from build123d import *

# Parameters (mm, degrees)
SKETCH_1_W          = 237
SKETCH_1_H          = 338
EXTRUDE_1_DEPTH     = 264
SKETCH_2_W          = 197
SKETCH_2_H          = 275
CUT_EXTRUDE_1_DEPTH = 248
SKETCH_3_W          = 237
SKETCH_3_H          = 5
EXTRUDE_2_DEPTH     = 255
EXTRUDE_START       = 70
SKETCH_4_R          = 5
EXTRUDE_3_DEPTH     = 30
SKETCH_6_W          = 338
SKETCH_6_H          = 237
EXTRUDE_6_DEPTH     = 34
FILLET_1_R          = 25
FILLET_2_R          = 10
FILLET_3_R          = 5
FILLET_4_R          = 15
FILLET_5_R          = 15


with BuildPart() as part:
    # 草图1 → 凸台-拉伸1 (new body)
    with BuildSketch(Plane.XY):
        Rectangle(SKETCH_1_W, SKETCH_1_H)
    extrude(amount=-EXTRUDE_1_DEPTH)

    # 草图2 → 切除-拉伸1 (cut)
    with BuildSketch(Plane.XY):
        Rectangle(SKETCH_2_W, SKETCH_2_H)
    extrude(amount=-CUT_EXTRUDE_1_DEPTH, mode=Mode.SUBTRACT)

    # 草图3 → 凸台-拉伸2 (add)
    with BuildSketch(Plane.XY):
        Rectangle(SKETCH_3_W, SKETCH_3_H)
    extrude(amount=-EXTRUDE_2_DEPTH)

    # 草图4 → 凸台-拉伸3 (add)
    with BuildSketch(Plane(origin=(0, 0, 0), x_dir=(1, 0, 0), z_dir=(0, 1, 0)).offset(EXTRUDE_START)):
        with Locations((118.5, 0)):
            Circle(SKETCH_4_R)
    extrude_3 = extrude(amount=EXTRUDE_3_DEPTH)

    # 镜向1: 凸台-拉伸3 across plane
    add(extrude_3.mirror(Plane.ZX))

    # 草图6 → 凸台-拉伸6 (add)
    with BuildSketch(Plane(origin=(59.25, 0, -59.25), x_dir=(0, 1, 0), z_dir=(-0.7071067811865438, 0, 0.7071067811865512))):
        with Locations((0, -200.292153571)):
            Rectangle(SKETCH_6_W, SKETCH_6_H)
    extrude(amount=-EXTRUDE_6_DEPTH)

    # 圆角1
    # the kernel refuses this fillet: 25 mm, written as the material it takes off along each edge
    with BuildSketch(Plane(origin=(118.5, -169, 59.671572875), x_dir=(-1, 0, 0), z_dir=(0, 0, -1))) as fillet_1_piece_1_section:
        with BuildLine():
            CenterArc((FILLET_1_R, FILLET_1_R), FILLET_1_R, 180, 90)
            Line((0, FILLET_1_R), (-FILLET_1_R * 0.02, FILLET_1_R))
            Line((-FILLET_1_R * 0.02, FILLET_1_R), (-FILLET_1_R * 0.02, -FILLET_1_R * 0.02))
            Line((-FILLET_1_R * 0.02, -FILLET_1_R * 0.02), (FILLET_1_R, -FILLET_1_R * 0.02))
            Line((FILLET_1_R, -FILLET_1_R * 0.02), (FILLET_1_R, 0))
        make_face()
    fillet_1_piece_1 = extrude(amount=323.671572875, mode=Mode.PRIVATE)
    fillet_1_piece_1 = split(fillet_1_piece_1, bisect_by=Plane(origin=(179.466338067, -163.404434067, -63.794765192), z_dir=(-0.7071067811865512, 0, -0.7071067811865438)), keep=Keep.TOP, mode=Mode.PRIVATE)
    add(fillet_1_piece_1, mode=Mode.SUBTRACT)
    with BuildSketch(Plane(origin=(-118.5, -169, 0), x_dir=(1, 0, 0), z_dir=(0, 0, -1)), Plane(origin=(-118.5, 169, 0), x_dir=(0, -1, 0), z_dir=(0, 0, -1))) as fillet_1_piece_2:
        with BuildLine():
            CenterArc((FILLET_1_R, -FILLET_1_R), FILLET_1_R, 90, 90)
            Line((0, -FILLET_1_R), (-FILLET_1_R * 0.02, -FILLET_1_R))
            Line((-FILLET_1_R * 0.02, -FILLET_1_R), (-FILLET_1_R * 0.02, FILLET_1_R * 0.02))
            Line((-FILLET_1_R * 0.02, FILLET_1_R * 0.02), (FILLET_1_R, FILLET_1_R * 0.02))
            Line((FILLET_1_R, FILLET_1_R * 0.02), (FILLET_1_R, 0))
        make_face()
    extrude(amount=264, mode=Mode.SUBTRACT)
    with BuildSketch(Plane(origin=(118.5, 169, 59.671572875), x_dir=(0, -1, 0), z_dir=(0, 0, -1))) as fillet_1_piece_3_section:
        with BuildLine():
            CenterArc((FILLET_1_R, FILLET_1_R), FILLET_1_R, 180, 90)
            Line((0, FILLET_1_R), (-FILLET_1_R * 0.02, FILLET_1_R))
            Line((-FILLET_1_R * 0.02, FILLET_1_R), (-FILLET_1_R * 0.02, -FILLET_1_R * 0.02))
            Line((-FILLET_1_R * 0.02, -FILLET_1_R * 0.02), (FILLET_1_R, -FILLET_1_R * 0.02))
            Line((FILLET_1_R, -FILLET_1_R * 0.02), (FILLET_1_R, 0))
        make_face()
    fillet_1_piece_3 = extrude(amount=323.671572875, mode=Mode.PRIVATE)
    fillet_1_piece_3 = split(fillet_1_piece_3, bisect_by=Plane(origin=(179.466338067, 163.404434067, -63.794765192), z_dir=(-0.7071067811865512, 0, -0.7071067811865438)), keep=Keep.TOP, mode=Mode.PRIVATE)
    add(fillet_1_piece_3, mode=Mode.SUBTRACT)
    with BuildSketch(Plane(origin=(284.670093579, -169, 166.170093579), x_dir=(-0.7071067811865512, -1.1368683772161603e-15, -0.7071067811865439), z_dir=(0.7071067811865438, 0, -0.7071067811865512))) as fillet_1_piece_4:
        with BuildLine():
            CenterArc((FILLET_1_R, FILLET_1_R), FILLET_1_R, 180, 90)
            Line((0, FILLET_1_R), (-FILLET_1_R * 0.02, FILLET_1_R))
            Line((-FILLET_1_R * 0.02, FILLET_1_R), (-FILLET_1_R * 0.02, -FILLET_1_R * 0.02))
            Line((-FILLET_1_R * 0.02, -FILLET_1_R * 0.02), (FILLET_1_R, -FILLET_1_R * 0.02))
            Line((FILLET_1_R, -FILLET_1_R * 0.02), (FILLET_1_R, 0))
        make_face()
    extrude(amount=34, mode=Mode.SUBTRACT)
    with BuildSketch(Plane(origin=(74.305826176, -169, 41.365746699), x_dir=(0.7071067811865512, 0, 0.7071067811865439), z_dir=(0.7071067811865438, 0, -0.7071067811865512))) as fillet_1_piece_5_section:
        with BuildLine():
            CenterArc((FILLET_1_R, -FILLET_1_R), FILLET_1_R, 90, 90)
            Line((0, -FILLET_1_R), (-FILLET_1_R * 0.02, -FILLET_1_R))
            Line((-FILLET_1_R * 0.02, -FILLET_1_R), (-FILLET_1_R * 0.02, FILLET_1_R * 0.02))
            Line((-FILLET_1_R * 0.02, FILLET_1_R * 0.02), (FILLET_1_R, FILLET_1_R * 0.02))
            Line((FILLET_1_R, FILLET_1_R * 0.02), (FILLET_1_R, 0))
        make_face()
    fillet_1_piece_5 = extrude(amount=94.5, mode=Mode.PRIVATE)
    fillet_1_piece_5 = split(fillet_1_piece_5, bisect_by=Plane(origin=(118.5, -163.795791277, -7.320817928), z_dir=(1, 0, 0)), keep=Keep.TOP, mode=Mode.PRIVATE)
    add(fillet_1_piece_5, mode=Mode.SUBTRACT)
    with BuildSketch(Plane(origin=(74.305826176, 169, 41.365746699), x_dir=(0.7071067811865512, 0, 0.7071067811865438), z_dir=(0.7071067811865438, 0, -0.7071067811865512))) as fillet_1_piece_6_section:
        with BuildLine():
            CenterArc((FILLET_1_R, FILLET_1_R), FILLET_1_R, 180, 90)
            Line((0, FILLET_1_R), (-FILLET_1_R * 0.02, FILLET_1_R))
            Line((-FILLET_1_R * 0.02, FILLET_1_R), (-FILLET_1_R * 0.02, -FILLET_1_R * 0.02))
            Line((-FILLET_1_R * 0.02, -FILLET_1_R * 0.02), (FILLET_1_R, -FILLET_1_R * 0.02))
            Line((FILLET_1_R, -FILLET_1_R * 0.02), (FILLET_1_R, 0))
        make_face()
    fillet_1_piece_6 = extrude(amount=94.5, mode=Mode.PRIVATE)
    fillet_1_piece_6 = split(fillet_1_piece_6, bisect_by=Plane(origin=(118.5, 163.795791277, -7.320817928), z_dir=(1, 0, 0)), keep=Keep.TOP, mode=Mode.PRIVATE)
    add(fillet_1_piece_6, mode=Mode.SUBTRACT)
    with BuildSketch(Plane(origin=(284.670093579, 169, 166.170093579), x_dir=(-0.7071067811865512, -3.4106051316484808e-15, -0.7071067811865439), z_dir=(0.7071067811865438, 0, -0.7071067811865512))) as fillet_1_piece_7:
        with BuildLine():
            CenterArc((FILLET_1_R, -FILLET_1_R), FILLET_1_R, 90, 90)
            Line((0, -FILLET_1_R), (-FILLET_1_R * 0.02, -FILLET_1_R))
            Line((-FILLET_1_R * 0.02, -FILLET_1_R), (-FILLET_1_R * 0.02, FILLET_1_R * 0.02))
            Line((-FILLET_1_R * 0.02, FILLET_1_R * 0.02), (FILLET_1_R, FILLET_1_R * 0.02))
            Line((FILLET_1_R, FILLET_1_R * 0.02), (FILLET_1_R, 0))
        make_face()
    extrude(amount=34, mode=Mode.SUBTRACT)
    with BuildSketch(Plane(origin=(118.5, -169, 59.671572875), x_dir=(-1, 0, 0), z_dir=(0, 0, -1))) as fillet_1_piece_8a_section:
        with BuildLine():
            CenterArc((FILLET_1_R, FILLET_1_R), FILLET_1_R, 180, 90)
            Line((0, FILLET_1_R), (-FILLET_1_R * 0.02, FILLET_1_R))
            Line((-FILLET_1_R * 0.02, FILLET_1_R), (-FILLET_1_R * 0.02, -FILLET_1_R * 0.02))
            Line((-FILLET_1_R * 0.02, -FILLET_1_R * 0.02), (FILLET_1_R, -FILLET_1_R * 0.02))
            Line((FILLET_1_R, -FILLET_1_R * 0.02), (FILLET_1_R, 0))
        make_face()
    fillet_1_piece_8a = extrude(amount=323.671572875, mode=Mode.PRIVATE)
    fillet_1_piece_8a = split(fillet_1_piece_8a, bisect_by=Plane(origin=(99.013375852, -163.038214912, 16.658197024), z_dir=(0.7071067811865512, 0, 0.7071067811865438)), keep=Keep.TOP, mode=Mode.PRIVATE)
    with BuildSketch(Plane(origin=(74.305826176, -169, 41.365746699), x_dir=(0.7071067811865512, 0, 0.7071067811865439), z_dir=(0.7071067811865438, 0, -0.7071067811865512))) as fillet_1_piece_8b_section:
        with BuildLine():
            CenterArc((FILLET_1_R, -FILLET_1_R), FILLET_1_R, 90, 90)
            Line((0, -FILLET_1_R), (-FILLET_1_R * 0.02, -FILLET_1_R))
            Line((-FILLET_1_R * 0.02, -FILLET_1_R), (-FILLET_1_R * 0.02, FILLET_1_R * 0.02))
            Line((-FILLET_1_R * 0.02, FILLET_1_R * 0.02), (FILLET_1_R, FILLET_1_R * 0.02))
            Line((FILLET_1_R, FILLET_1_R * 0.02), (FILLET_1_R, 0))
        make_face()
    fillet_1_piece_8b = extrude(amount=94.5, mode=Mode.PRIVATE)
    fillet_1_piece_8b = split(fillet_1_piece_8b, bisect_by=Plane(origin=(118.5, -163.038214912, 24.729821031), z_dir=(-1, 0, 0)), keep=Keep.TOP, mode=Mode.PRIVATE)
    fillet_1_piece_8 = fillet_1_piece_8a & fillet_1_piece_8b
    add(fillet_1_piece_8, mode=Mode.SUBTRACT)
    with BuildSketch(Plane(origin=(118.5, 169, 59.671572875), x_dir=(0, -1, 0), z_dir=(0, 0, -1))) as fillet_1_piece_9a_section:
        with BuildLine():
            CenterArc((FILLET_1_R, FILLET_1_R), FILLET_1_R, 180, 90)
            Line((0, FILLET_1_R), (-FILLET_1_R * 0.02, FILLET_1_R))
            Line((-FILLET_1_R * 0.02, FILLET_1_R), (-FILLET_1_R * 0.02, -FILLET_1_R * 0.02))
            Line((-FILLET_1_R * 0.02, -FILLET_1_R * 0.02), (FILLET_1_R, -FILLET_1_R * 0.02))
            Line((FILLET_1_R, -FILLET_1_R * 0.02), (FILLET_1_R, 0))
        make_face()
    fillet_1_piece_9a = extrude(amount=323.671572875, mode=Mode.PRIVATE)
    fillet_1_piece_9a = split(fillet_1_piece_9a, bisect_by=Plane(origin=(99.013375852, 163.038214912, 16.658197024), z_dir=(0.7071067811865512, 0, 0.7071067811865438)), keep=Keep.TOP, mode=Mode.PRIVATE)
    with BuildSketch(Plane(origin=(74.305826176, 169, 41.365746699), x_dir=(0.7071067811865512, 0, 0.7071067811865438), z_dir=(0.7071067811865438, 0, -0.7071067811865512))) as fillet_1_piece_9b_section:
        with BuildLine():
            CenterArc((FILLET_1_R, FILLET_1_R), FILLET_1_R, 180, 90)
            Line((0, FILLET_1_R), (-FILLET_1_R * 0.02, FILLET_1_R))
            Line((-FILLET_1_R * 0.02, FILLET_1_R), (-FILLET_1_R * 0.02, -FILLET_1_R * 0.02))
            Line((-FILLET_1_R * 0.02, -FILLET_1_R * 0.02), (FILLET_1_R, -FILLET_1_R * 0.02))
            Line((FILLET_1_R, -FILLET_1_R * 0.02), (FILLET_1_R, 0))
        make_face()
    fillet_1_piece_9b = extrude(amount=94.5, mode=Mode.PRIVATE)
    fillet_1_piece_9b = split(fillet_1_piece_9b, bisect_by=Plane(origin=(118.5, 163.038214912, 24.729821031), z_dir=(-1, 0, 0)), keep=Keep.TOP, mode=Mode.PRIVATE)
    fillet_1_piece_9 = fillet_1_piece_9a & fillet_1_piece_9b
    add(fillet_1_piece_9, mode=Mode.SUBTRACT)

    # 圆角2
    fillet_2_edges = [part.edges().sort_by_distance(p)[0] for p in [
        (0, -169, -264),
        (118.5, 0, -264),
        (-118.5, 0, -264),
        (0, 169, -264),
        (-111.17766953, 161.67766953, -264),
        (111.17766953, 161.67766953, -264),
        (-111.17766953, -161.67766953, -264),
        (111.17766953, -161.67766953, -264),
    ]]
    fillet(fillet_2_edges, radius=FILLET_2_R)

    # 圆角3
    fillet_3_edges = [part.edges().sort_by_distance(p)[0] for p in [
        (224.919570569, -169, 58.336309448),
        (141.127416998, 0, -25.455844123),
        (224.919570569, 169, 58.336309448),
        (308.711724139, 0, 142.128463018),
        (146.305086528, 161.67766953, -20.278174593),
        (303.53405461, 161.67766953, 136.950793489),
        (303.53405461, -161.67766953, 136.950793489),
        (146.305086528, -161.67766953, -20.278174593),
    ]]
    fillet(fillet_3_edges, radius=FILLET_3_R)

    # 圆角4
    fillet_4_edges = [part.edges().sort_by_distance(p)[0] for p in [
        (98.5, -70, -248),
        (98.5, 137.5, -124),
        (0, -137.5, -248),
        (98.5, -137.5, -124),
        (-98.5, -137.5, -124),
        (0, 137.5, -248),
        (-98.5, 137.5, -124),
        (-98.5, -70, -248),
    ]]
    fillet(fillet_4_edges, radius=FILLET_4_R)

    # 圆角5
    # the kernel refuses this fillet: 15 mm, written as the material it adds along each edge
    with BuildSketch(Plane(origin=(-83.5, 122.5, -233), x_dir=(0, 0, -1), z_dir=(-1, 0, 0))) as fillet_5_piece_1_section:
        Polygon((0, 0), (FILLET_5_R * 1.02, 0), (FILLET_5_R * 1.02, -FILLET_5_R * 1.02), (0, -FILLET_5_R * 1.02), align=None)
    fillet_5_piece_1 = extrude(amount=FILLET_5_R * 1.02, mode=Mode.PRIVATE)
    fillet_5_piece_1 = fillet_5_piece_1 - Plane(origin=(-83.5, 122.5, -233), x_dir=(0, -0.7071067811865475, 0.7071067811865475), z_dir=(-1, 0, 0)) * Sphere(FILLET_5_R, mode=Mode.PRIVATE)
    add(fillet_5_piece_1)
    with BuildSketch(Plane(origin=(83.5, 122.5, -233), x_dir=(0, 0, -1), z_dir=(1, 0, 0))) as fillet_5_piece_2_section:
        Polygon((0, 0), (FILLET_5_R * 1.02, 0), (FILLET_5_R * 1.02, FILLET_5_R * 1.02), (0, FILLET_5_R * 1.02), align=None)
    fillet_5_piece_2 = extrude(amount=FILLET_5_R * 1.02, mode=Mode.PRIVATE)
    fillet_5_piece_2 = fillet_5_piece_2 - Plane(origin=(83.5, 122.5, -233), x_dir=(0, -0.7071067811865475, 0.7071067811865475), z_dir=(1, 0, 0)) * Sphere(FILLET_5_R, mode=Mode.PRIVATE)
    add(fillet_5_piece_2)
    with BuildSketch(Plane(origin=(-98.5, -35, -248), x_dir=(0, 0, 1), z_dir=(0, 1, 0)), Plane(origin=(98.5, 122.5, -248), x_dir=(0, 0, 1), z_dir=(0, -1, 0))) as fillet_5_piece_3:
        with BuildLine():
            CenterArc((FILLET_5_R, FILLET_5_R), FILLET_5_R, 180, 90)
            Line((0, FILLET_5_R), (0, 0))
            Line((0, 0), (FILLET_5_R, 0))
        make_face()
    extrude(amount=157.5)


solid = part.part
Input: part model. Units: mm. Frame: model coordinates. A direction names the side the tool comes from. Round coordinates to 2 decimals unless told otherwise and drop trailing zeros. Order: outer loops, then holes, each group sorted by start corner. A loop starts at its lowest first (then second) coordinate and runs counter-clockwise, first axis right, second up. Notation, with made-up numbers: (-36.75, -4) - (-17.75, -4) arc R28 cw to (-17.75, 14) - close; hole circle Ø10 at (83.25, 45). An arc over 180 degrees is marked (long way). Use a Markdown table: item, result.
1. Section B-B on y = -10. Return the cut outline in (x, z), then the cut area to 3 significant figures.
Evaluation:
| item | result |
|---|---|
| outline | (-118.5, -254) arc R10 ccw to (-108.5, -264) - (108.5, -264) arc R10 ccw to (118.5, -254) - (118.5, -2.83) - (137.59, -21.92) arc R5 ccw to (144.66, -21.92) - (305.18, 138.59) arc R5 ccw to (305.18, 145.66) - (284.67, 166.17) - (118.5, 0) - (98.5, 0) - (98.5, -233) arc R15 cw to (83.5, -248) - (-83.5, -248) arc R15 cw to (-98.5, -233) - (-98.5, 0) - (-118.5, 0) - close |
| area | 21,800 mm^2 |
2. Access query for faces 1 (the face through (-93.99, 133.22, -118.13)), 2 (the face through (289.464, 161.871, 150.745)). Directions: +Z, -Z, +X, -X, +Y, -Y. A direction counts if a zero-diameter tool reaches every point of the face in a straight line with its end or side. Return the directions, or none.
Evaluation:
| item | result |
|---|---|
| face 1 | +Z |
| face 2 | +Z, +X, +Y |
3. Section C-C on x = -52. Return the cut outline in (y, z).
Evaluation:
| item | result |
|---|---|
| outline | (-169, -254) arc R10 ccw to (-159, -264) - (159, -264) arc R10 ccw to (169, -254) - (169, 0) - (137.5, 0) - (137.5, -233) arc R15 cw to (122.5, -248) - (2.5, -248) - (2.5, 0) - (-2.5, 0) - (-2.5, -248) - (-122.5, -248) arc R15 cw to (-137.5, -233) - (-137.5, 0) - (-169, 0) - close |
4. Section D-D on y = 89. Return the cut outline in (x, z).
Evaluation:
| item | result |
|---|---|
| outline | (-118.5, -254) arc R10 ccw to (-108.5, -264) - (108.5, -264) arc R10 ccw to (118.5, -254) - (118.5, -5) arc R5 ccw to (120.33, -4.65) - (137.59, -21.92) arc R5 ccw to (144.66, -21.92) - (305.18, 138.59) arc R5 ccw to (305.18, 145.66) - (284.67, 166.17) - (122.04, 3.54) arc R5 ccw to (113.5, 0) - (98.5, 0) - (98.5, -233) arc R15 cw to (83.5, -248) - (-83.5, -248) arc R15 cw to (-98.5, -233) - (-98.5, 0) - (-118.5, 0) - close |
5. First-contact query: pin 1 (5 mm diameter, centred on y = 76, z = -86.5, fed in from +X); pin 2 (5 mm diameter, centred on x = -45.5, y = -119, fed in from +Z); pin 3 (4 mm diameter, centred on x = 116, z = 3, fed in from +Y). Flat tips, straight axial feed; report the tip coordinate or a pass-through.
Evaluation:
| item | result |
|---|---|
| pin 1 | x = 118.5 |
| pin 2 | z = -248 |
| pin 3 | y = 100 |
6. Material intervals for probe 1 along Y at (x, z) = (-2.5, -224); probe 2 along X at (y, z) = (-115, -194); probe 3 along X at (y, z) = (141.5, -26), sorted ascending.
Evaluation:
| item | result |
|---|---|
| probe 1 | -169 to -137.5, -2.5 to 2.5, 137.5 to 169 |
| probe 2 | -118.5 to -98.5, 98.5 to 118.5 |
| probe 3 | -118.5 to 118.5 |
7. Section A-A on z = -148.5. Return the cut outline in (x, y).
Evaluation:
| item | result |
|---|---|
| outline | (-118.5, -144) arc R25 ccw to (-93.5, -169) - (93.5, -169) arc R25 ccw to (118.5, -144) - (118.5, 144) arc R25 ccw to (93.5, 169) - (-93.5, 169) arc R25 ccw to (-118.5, 144) - close; hole (-98.5, -122.5) arc R15 ccw to (-83.5, -137.5) - (83.5, -137.5) arc R15 ccw to (98.5, -122.5) - (98.5, -2.5) - (-98.5, -2.5) - close; hole (-98.5, 2.5) - (98.5, 2.5) - (98.5, 122.5) arc R15 ccw to (83.5, 137.5) - (-83.5, 137.5) arc R15 ccw to (-98.5, 122.5) - close |
8. Mould query, pull axis X, two halves, no side actions, for faces 3 (the face through (289.74, -161.48, 151.02)), 4 (the face through (1.17, -133.22, -243.49)), 5 (the face through (-2, 2, 0)). Classes: +X half, -X half, draft (parallel to the pull), parting line (faces both ways), or undercut.
Evaluation:
| item | result |
|---|---|
| face 3 | +X half |
| face 4 | undercut |
| face 5 | draft |
